Geometry check sheet. Reference: drawing and pictorial views, mm from the part's lowest x, y, z. A direction names the side the tool comes from. Give positions to 0.01 mm unless a question says otherwise; leave off trailing zeros. Order: outer loops, then holes, each group sorted by start corner. A loop starts at its lowest first (then second) coordinate and runs counter-clockwise, first axis right, second up. Notation, with made-up numbers: (-34.5, -5.75) - (-12.5, -5.75) arc R11 cw to (-12.5, 6.25) - close; hole circle Ø7 at (-30.75, -9.75). An arc over 180 degrees is marked (long way). Answer as a JSON object with one key per item and string values.
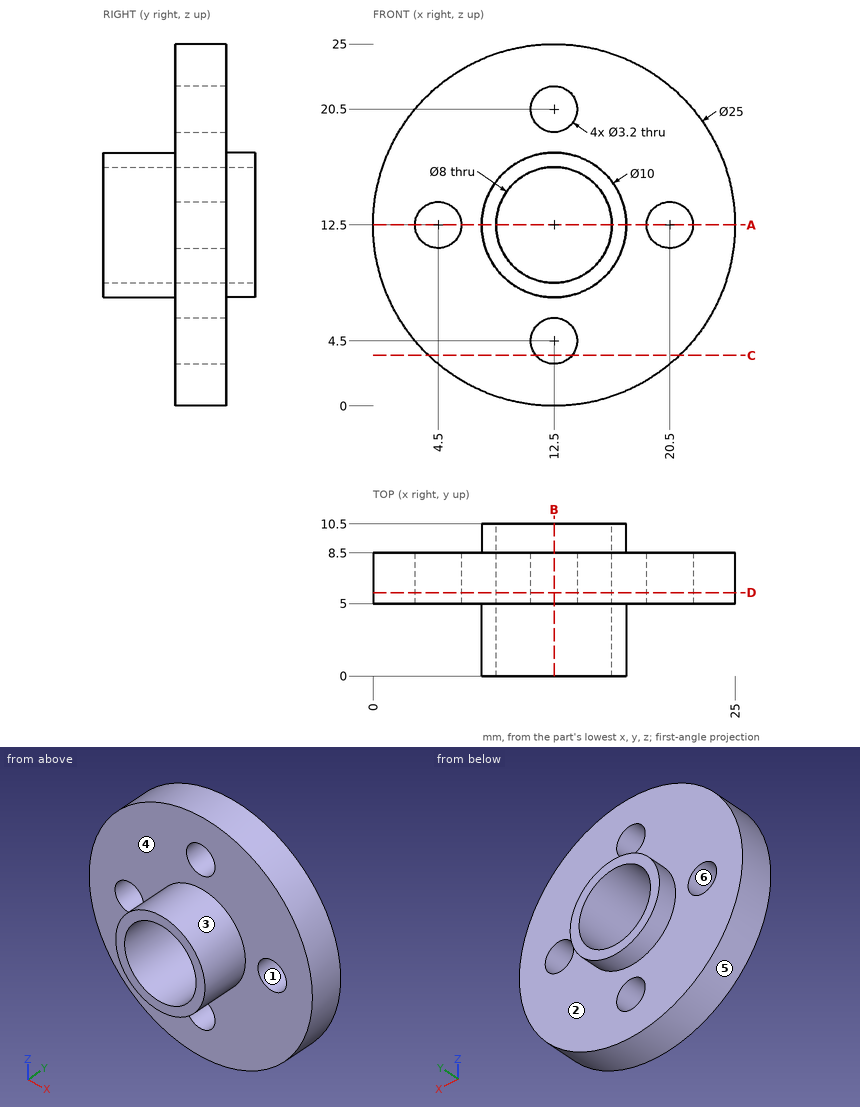
(1) Release check for a two-part mould opening along Z. For the marked faces 4, 5 and 6 record: pulls with the +Z half, pulls with the -Z half, needs draft (parallel to the pull), parting line crosses it, or undercut.
Computed values:
{"face 4": "needs draft", "face 5": "parting line crosses it", "face 6": "undercut"}
(2) Section check B-B (x = 12.5). Record the cut outline in (y, z), then the cut area to 3 significant figures.
Computed values:
{"outline": "(0, 7.5) - (5, 7.5) - (5, 6.1) - (8.5, 6.1) - (8.5, 7.5) - (10.5, 7.5) - (10.5, 8.5) - (0, 8.5) - close; (0, 16.5) - (10.5, 16.5) - (10.5, 17.5) - (8.5, 17.5) - (8.5, 18.9) - (5, 18.9) - (5, 17.5) - (0, 17.5) - close; (5, 0) - (8.5, 0) - (8.5, 2.9) - (5, 2.9) - close; (5, 22.1) - (8.5, 22.1) - (8.5, 25) - (5, 25) - close", "area": "51.1 mm²"}
(3) Access from +Z, -Z, +X, -X, +Y, -Y to the whole of each face (thin tool, end or side, straight path). Record for the marked faces 1, 2 and 3.
Computed values:
{"face 1": "+Y, -Y", "face 2": "+Y", "face 3": "-Y"}
(4) Section check A-A (z = 12.5). Record the cut outline in (x, y), then the cut area to 3 significant figures.
Computed values:
{"outline": "(0, 5) - (2.9, 5) - (2.9, 8.5) - (0, 8.5) - close; (6.1, 5) - (7.5, 5) - (7.5, 0) - (8.5, 0) - (8.5, 10.5) - (7.5, 10.5) - (7.5, 8.5) - (6.1, 8.5) - close; (16.5, 0) - (17.5, 0) - (17.5, 5) - (18.9, 5) - (18.9, 8.5) - (17.5, 8.5) - (17.5, 10.5) - (16.5, 10.5) - close; (22.1, 5) - (25, 5) - (25, 8.5) - (22.1, 8.5) - close", "area": "51.1 mm²"}
(5) Gauge pin test, flat ends, axial feed: pin 1 Ø1.5 at (y, z) = (9, 21.5) entering from -X; pin 2 Ø1 at (x, z) = (15, 3) entering from -Y; pin 3 Ø1 at (y, z) = (8.5, 18) entering from +X; pin 4 Ø7.5 at (x, z) = (8.5, 17) entering from +Y. Record the tip position at first contact, or that the pin passes through.
Computed values:
{"pin 1": "stops at x = 3.28", "pin 2": "stops at y = 5", "pin 3": "stops at x = 23.96", "pin 4": "stops at y = 10.5"}
(6) Material ranges on line 1 along Z through (x, y) = (12.5, 6.3); line 2 along Z through (x, y) = (12.5, 3), recorded low to high. Write a range as [from, to].
Computed values:
{"line 1": "z = [0, 2.9], [6.1, 8.5], [16.5, 18.9], [22.1, 25]", "line 2": "z = [7.5, 8.5], [16.5, 17.5]"}
(7) Section check D-D (y = 5.75). Record the cut outline in (x, z).
Computed values:
{"outline": "circle Ø25 at (12.5, 12.5); hole circle Ø3.2 at (4.5, 12.5); hole circle Ø8 at (12.5, 12.5); hole circle Ø3.2 at (12.5, 4.5); hole circle Ø3.2 at (12.5, 20.5); hole circle Ø3.2 at (20.5, 12.5)"}
(8) Section check C-C (z = 3.5). Record the cut outline in (x, y).
Computed values:
{"outline": "(3.83, 5) - (11.25, 5) - (11.25, 8.5) - (3.83, 8.5) - close; (13.75, 5) - (21.17, 5) - (21.17, 8.5) - (13.75, 8.5) - close"}
